```python
from build123d import *

# Parameters (mm, degrees)
BOSS_EXTRUDE1_DEPTH = 2.5
FILLET1_R           = 8
FILLET2_R           = 8


with BuildPart() as part:
    # Sketch1 → Boss-Extrude1 (new body)
    with BuildSketch(Plane.XY):
        Polygon((19.5, -53), (25, -53), (25, 53), (-25, 53), (-25, -53), (-19.5, -53), (-19.5, -47.017253966), (19.5, -47.017253966), align=None)
    extrude(amount=BOSS_EXTRUDE1_DEPTH)

    # Fillet1
    fillet1_edges = [part.edges().sort_by_distance(p)[0] for p in [
        (-25, 53, 1.25),
        (25, 53, 1.25),
    ]]
    fillet(fillet1_edges, radius=FILLET1_R)

    # Fillet2
    # the kernel refuses this fillet: 8 mm, written as the material it takes off along each edge
    with BuildSketch(Plane(origin=(-25, 45, 0), x_dir=(1, 0, 0), z_dir=(0, -1, 0))) as fillet2_piece_1:
        with BuildLine():
            CenterArc((5.809475019, 8), FILLET2_R, 223.432536558, 46.567463442)
            Line((0, 2.5), (-0.1161895, 2.39))
            ThreePointArc((-0.1161895, 2.39), (-0.16, 1.25), (-0.16, 0))
            Line((-0.16, 0), (0, -0.16))
            Line((0, -0.16), (5.809475019, -0.16))
            Line((5.809475019, -0.16), (5.809475019, 0))
        make_face()
    extrude(amount=112.523687548, mode=Mode.SUBTRACT)
    with BuildSketch(Plane(origin=(-17, 45, 0), x_dir=(0, 1, 0), z_dir=(1, 0, 0))) as fillet2_piece_2:
        with BuildLine():
            CenterArc((2.190524981, 8), FILLET2_R, 270, 46.567463442)
            Line((8, 2.5), (8.1161895, 2.39))
            ThreePointArc((8.1161895, 2.39), (8.16, 1.25), (8.16, 0))
            Line((8.16, 0), (8, -0.16))
            Line((8, -0.16), (2.190524981, -0.16))
            Line((2.190524981, -0.16), (2.190524981, 0))
        make_face()
    revolve(axis=Axis((-17, 45, 0), (0, 0, 1)), revolution_arc=90, mode=Mode.SUBTRACT)
    with BuildSketch(Plane(origin=(17, 53, 0), x_dir=(0, -1, 0), z_dir=(-1, 0, 0))) as fillet2_piece_3:
        with BuildLine():
            CenterArc((5.809475019, 8), FILLET2_R, 223.432536558, 46.567463442)
            Line((0, 2.5), (-0.1161895, 2.39))
            ThreePointArc((-0.1161895, 2.39), (-0.16, 1.25), (-0.16, 0))
            Line((-0.16, 0), (0, -0.16))
            Line((0, -0.16), (5.809475019, -0.16))
            Line((5.809475019, -0.16), (5.809475019, 0))
        make_face()
    extrude(amount=34, mode=Mode.SUBTRACT)
    with BuildSketch(Plane(origin=(17, 45, 0), x_dir=(1, 0, 0), z_dir=(0, -1, 0))) as fillet2_piece_4:
        with BuildLine():
            CenterArc((2.190524981, 8), FILLET2_R, 270, 46.567463442)
            Line((8, 2.5), (8.1161895, 2.39))
            ThreePointArc((8.1161895, 2.39), (8.16, 1.25), (8.16, 0))
            Line((8.16, 0), (8, -0.16))
            Line((8, -0.16), (2.190524981, -0.16))
            Line((2.190524981, -0.16), (2.190524981, 0))
        make_face()
    revolve(axis=Axis((17, 45, 0), (0, 0, 1)), revolution_arc=90, mode=Mode.SUBTRACT)
    with BuildSketch(Plane(origin=(25, -67.523687548, 0), x_dir=(0, 0, 1), z_dir=(0, 1, 0))) as fillet2_piece_5:
        with BuildLine():
            CenterArc((8, -5.809475019), FILLET2_R, 133.432536558, 46.567463442)
            Line((0, -5.809475019), (-0.16, -5.809475019))
            Line((-0.16, -5.809475019), (-0.16, 0))
            Line((-0.16, 0), (0, 0.16))
            ThreePointArc((0, 0.16), (1.25, 0.16), (2.39, 0.1161895))
            Line((2.39, 0.1161895), (2.5, 0))
        make_face()
    extrude(amount=112.523687548, mode=Mode.SUBTRACT)


solid = part.part
```
Could you check a few things on this model? Use its own coordinates, in mm. A direction names the side the tool comes from. Coordinates: 2 decimals unless noted, no trailing zeros. Loops run counter-clockwise (first coordinate to the right, second up) from the corner with the lowest first, then second, coordinate; pieces in that order, holes last.
1) Will these pins go through, and if not, where does the flat tip stop? pin 1 Ø0.8 at (x, z) = (-9, 1) entering from -Y; pin 2 Ø1.5 at (y, z) = (-21, 2) entering from -X.
Reported:
pin 1: stops at y = -47.02
pin 2: stops at x = -25
2) Thinking about a two-plate mould opening in X: for faces 3 (the face through (-19.5, -50, 1)), 4 (the face through (-22.395, -3.314, 0.67)), 5 (the face through (-22, -53, 2)), which applies, released by +X, released by -X, zero draft, split by the parting line, or undercut?
Reported:
face 3: undercut
face 4: released by -X
face 5: zero draft
3) Which directions (+Z, -Z, +X, -X, +Y, -Y) give clear straight access to the entire face, cutting with the end or side of a thin tool? Please do faces 1 (the face through (22, -53, 2)), 2 (the face through (19.5, -50, 1)).
Reported:
face 1: +Z, -Z, +X, -X, -Y
face 2: +Z, -Z, -Y
4) Please list where these lines run through material, in increasing order: line 1 along Z through (x, y) = (-21.5, -32); line 2 along Y through (x, z) = (-15.5, 1.3); line 3 along X through (y, z) = (29, 0.8).
Reported:
line 1: z = 0.34 to 2.5
line 2: y = -47.02 to 51.56
line 3: x = -22.68 to 22.68
5) Imagine slicing it at A-A (x = -11). List the corners of the cut face in (y, z) for me.
Reported:
outline: (-47.02, 0) - (47.19, 0) arc R8 ccw to (53, 2.5) - (-47.02, 2.5) - close
6) Imagine slicing it at B-B (y = -24). List the corners of the cut face in (x, z) for me.
Reported:
outline: (-25, 2.5) arc R8 ccw to (-19.19, 0) - (19.19, 0) arc R8 ccw to (25, 2.5) - close
